```python
from build123d import *

# Parameters (mm, degrees)
ESQUISSE1_W             = 50
ESQUISSE1_H             = 460
BOSS_EXTRU_1_DEPTH      = 3
ESQUISSE2_W             = 20
ESQUISSE2_H             = 25
ENL_V_MAT_EXTRU_2_DEPTH = 232.37415586
ESQUISSE5_W             = 25
ESQUISSE5_H             = 20
BOSS_EXTRU_3_DEPTH      = 3


with BuildPart() as part:
    # Esquisse1 → Boss.-Extru.1 (new body)
    with BuildSketch(Plane(origin=(0, 0, 0), x_dir=(0, 0, -1), z_dir=(1, 0, 0))):
        Rectangle(ESQUISSE1_W, ESQUISSE1_H)
    extrude(amount=BOSS_EXTRU_1_DEPTH)

    # Esquisse2 → Enlèv. mat.-Extru.2 (cut, through all)
    with BuildSketch(Plane(origin=(3, 0, 0), x_dir=(0, 0, -1), z_dir=(1, 0, 0))):
        with Locations((15, -205)):
            Rectangle(ESQUISSE2_W, ESQUISSE2_H)
    extrude(amount=-ENL_V_MAT_EXTRU_2_DEPTH, mode=Mode.SUBTRACT)

    # Esquisse5 → Boss.-Extru.3 (add)
    with BuildSketch(Plane(origin=(3, 0, 0), x_dir=(0, 0, -1), z_dir=(1, 0, 0))):
        with Locations((0, 240)):
            Rectangle(ESQUISSE5_W, ESQUISSE5_H)
    extrude(amount=-BOSS_EXTRU_3_DEPTH)


solid = part.part
```
The listing builds one solid part. Answer for the finished solid, in the listing's coordinates (mm). Round coordinates to 2 decimals unless told otherwise and drop trailing zeros. Order: outer loops, then holes, each group sorted by start corner. A loop starts at its lowest first (then second) coordinate and runs counter-clockwise, first axis right, second up. Notation, with made-up numbers: (6.5, 32) - (30.5, 32) arc R16 ccw to (30.5, 43) - close; hole circle Ø2 at (-30.5, 66). An arc over 180 degrees is marked (long way). Put each result on its own line as item: value. Start each with the question number.
(1) Find section A-A (x = 1.8). Give the vertices of the cut face in (y, z), plus the area to 3 significant figures.
(2) Straight lines are drawn through the part: probe 1 along Y at (x, z) = (1, -15); probe 2 along Y at (x, z) = (2.55, 17); probe 3 along Z at (x, y) = (1.9, -206). For each, find the intervals that lie inside material, in ascending order. Write a range as from..to.
(3) Given P1, Ø1.5, axis at x = 1, z = -16, coming from the +Y side; P2, Ø0.9, axis at x = 1.5, y = 241, coming from the +Z side, each flat-ended and moving along its own axis, determine where each tip first touches the part or whether it passes through.
(4) Find section B-B (z = 17). Give the vertices of the cut face in (x, y).
Reply:
1. outline: (-230, -25) - (-217.5, -25) - (-217.5, -5) - (-192.5, -5) - (-192.5, -25) - (230, -25) - (230, -12.5) - (250, -12.5) - (250, 12.5) - (230, 12.5) - (230, 25) - (-230, 25) - close
1. area: 23,000 mm^2
2. probe 1: -230..-217.5, -192.5..230
2. probe 2: -230..230
2. probe 3: -5..25
3. P1: y = 230
3. P2: z = 12.5
4. outline: (0, -230) - (3, -230) - (3, 230) - (0, 230) - close
